Geometry check sheet. Reference: the model listing, model coordinates, mm. Face numbers are marked on the shaded views. A direction names the side the tool comes from. Coordinates: 2 decimals unless noted, no trailing zeros. Loops run counter-clockwise (first coordinate to the right, second up) from the corner with the lowest first, then second, coordinate; pieces in that order, holes last.
from build123d import *

# Parameters (mm, degrees)
F1_DEPTH = 63.5
F2_DEPTH = 12.7
F0_W     = 23.580307
F0_H     = 19.05
F3_DEPTH = 25.4
F0_W_2   = 25.4
F0_H_2   = 28.575


with BuildPart() as f1:
    # F0 (on Front) → F1 (new body, symmetric)
    with BuildSketch(Plane.XZ):
        Polygon((41.275, -9.525), (41.275, 9.525), (22.225, 9.525), (-41.275, 9.525), (-41.275, -9.525), align=None)
    extrude(amount=F1_DEPTH, both=True)

    # F0 (on Front) → F2 (join, symmetric)
    with BuildSketch(Plane.XZ):
        with BuildLine():
            Line((-41.275, 9.525), (22.225, 9.525))
            Line((22.225, 9.525), (22.225, 27.0002))
            ThreePointArc((22.225, 27.0002), (32.454296, 51.695904), (57.15, 61.9252))
            add(Edge.make_bspline(
                [(-41.275, 9.525), (0.105267, 11.943228), (14.862967, 64.384811), (57.15, 61.9252)],
                knots=[0, 0, 0, 0, 111.504536, 111.504536, 111.504536, 111.504536], degree=3))
        make_face()
    extrude(amount=F2_DEPTH, both=True)

    # F0 (on Front) → F3 (join, symmetric)
    with BuildSketch(Plane.XZ):
        with BuildLine():
            Line((22.225, 9.525), (41.275, 9.525))
            Line((41.275, 9.525), (41.275, 27.0002))
            ThreePointArc((41.275, 27.0002), (45.92468, 38.22552), (57.15, 42.8752))
            Line((57.15, 42.8752), (60.325, 42.8752))
            Line((60.325, 42.8752), (60.325, 61.9252))
            Line((60.325, 61.9252), (57.15, 61.9252))
            ThreePointArc((57.15, 61.9252), (32.454296, 51.695904), (22.225, 27.0002))
            Line((22.225, 27.0002), (22.225, 9.525))
        make_face()
        with Locations((72.115153, 52.4002)):
            Rectangle(F0_W, F0_H)
    extrude(amount=F3_DEPTH, both=True)

    # F0 (on Front) → F4 (revolve)
    with BuildSketch(Plane.XZ):
        with Locations((98.425, 50.186728)):
            Rectangle(F0_W_2, F0_H_2)
    revolve(axis=Axis((85.725, 0, 50.186728), (0, 0, -1)))


solid = f1.part
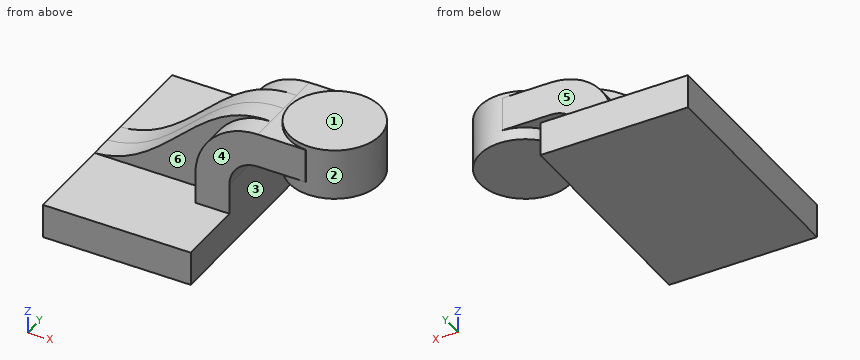
(1) Access from +Z, -Z, +X, -X, +Y, -Y to the whole of each face (thin tool, end or side, straight path). Record for the marked faces 4, 5 and 6.
Findings:
face 4: +Z, +X, -X, -Y
face 5: +Z, +X, -X, +Y
face 6: +Z, -X, -Y
(2) Gauge pin test, flat ends, axial feed: pin 1 Ø4 at (y, z) = (16, 20.5) entering from -X (3 decimals); pin 2 Ø2 at (x, z) = (77.5, 38.5) entering from +Y; pin 3 Ø18.5 at (y, z) = (23.5, 3) entering from +X (3 decimals). Record the tip position at first contact, or that the pin passes through.
Findings:
pin 1: stops at x = 22.225
pin 2: stops at y = 24.35
pin 3: stops at x = 41.275
(3) Sectioned sample at D-D on y = -32. Record the cut outline in (x, z) (3 decimals).
Findings:
outline: (-41.275, -9.525) - (41.275, -9.525) - (41.275, 9.525) - (-41.275, 9.525) - close
(4) Sectioned sample at B-B on y = -18.5. Record the cut outline in (x, z) (3 decimals), and give its area (3 significant figures).
Findings:
outline: (-41.275, -9.525) - (41.275, -9.525) - (41.275, 27) arc R15.875 cw to (57.15, 42.875) - (68.321, 42.875) - (68.321, 35.899) - (103.129, 35.899) - (103.129, 64.474) - (68.321, 64.474) - (68.321, 61.925) - (57.15, 61.925) arc R34.925 ccw to (22.225, 27) - (22.225, 9.525) - (-41.275, 9.525) - close
area: 3,870 mm2
(5) Sectioned sample at A-A on y = 15.5. Record the cut outline in (x, z) (3 decimals), and give its area (3 significant figures).
Findings:
outline: (-41.275, -9.525) - (41.275, -9.525) - (41.275, 27) arc R15.875 cw to (57.15, 42.875) - (65.603, 42.875) - (65.603, 35.899) - (105.847, 35.899) - (105.847, 64.474) - (65.603, 64.474) - (65.603, 61.925) - (57.15, 61.925) arc R34.925 ccw to (22.225, 27) - (22.225, 9.525) - (-41.275, 9.525) - close
area: 3,980 mm2
(6) Sectioned sample at C-C on x = 97.5. Record the cut outline in (y, z), and give its area (3 significant figures).
Findings:
outline: (-22.51, 35.9) - (22.51, 35.9) - (22.51, 64.47) - (-22.51, 64.47) - close
area: 1,290 mm2
(7) Draft check along X on the marked faces 1, 2 and 3. Enter one of: +X half, -X half, draft (parallel to the pull), parting line (faces both ways), or undercut.
Findings:
face 1: draft
face 2: undercut
face 3: +X half
(8) Scan lines: L1, parallel to Z at x = -32, y = -31 (3 decimals); L2, parallel to Y at x = 56.5, z = 48.5; L3, parallel to X at y = 1, z = 5 (3 decimals). Record each from-to range of solid material in increasing order.
Findings:
L1: z = -9.525 to 9.525
L2: y = -25.4 to 25.4
L3: x = -41.275 to 41.275
